```python
from build123d import *

# Parameters (mm, degrees)
SKETCH1_W           = 18
SKETCH1_H           = 13
SKETCH1_R           = 0.5
SKETCH1_R_2         = 1.5
BOSS_EXTRUDE1_DEPTH = 1.5
SKETCH2_W           = 1.829914293
SKETCH2_H           = 3.482740107
BOSS_EXTRUDE2_DEPTH = 1.75
SKETCH3_W           = 4.928962693
SKETCH3_H           = 2.951474666
SKETCH3_W_2         = 1.003501387
SKETCH3_H_2         = 2.331664987
SKETCH3_W_3         = 0.8854424
SKETCH3_W_4         = 0.944471893
SKETCH3_H_3         = 2.095547014
SKETCH3_W_5         = 0.914957147
SKETCH3_H_4         = 2.213606
SKETCH3_W_6         = 2.420209226
SKETCH3_H_5         = 0.914957147
SKETCH3_W_7         = 2.331664986
SKETCH3_W_8         = 2.066032267
SKETCH3_W_9         = 0.79689816
SKETCH3_W_10        = 2.774386186
SKETCH3_H_6         = 2.184091253
SKETCH3_W_11        = 1.741370054
SKETCH3_W_12        = 1.534766827
BOSS_EXTRUDE3_DEPTH = 0.75


with BuildPart() as part:
    # Sketch1 → Boss-Extrude1 (new body)
    with BuildSketch(Plane(origin=(0, 0, 0), x_dir=(1, 0, 0), z_dir=(0, 1, 0))):
        with Locations((9, -6.5)):
            Rectangle(SKETCH1_W, SKETCH1_H)
        with Locations((1.38, -1.38)):
            Circle(SKETCH1_R, mode=Mode.SUBTRACT)
        with Locations((3.92, -1.38)):
            Circle(SKETCH1_R, mode=Mode.SUBTRACT)
        with Locations((6.46, -1.38)):
            Circle(SKETCH1_R, mode=Mode.SUBTRACT)
        with Locations((9, -1.38)):
            Circle(SKETCH1_R, mode=Mode.SUBTRACT)
        with Locations((11.54, -1.38)):
            Circle(SKETCH1_R, mode=Mode.SUBTRACT)
        with Locations((14.08, -1.38)):
            Circle(SKETCH1_R, mode=Mode.SUBTRACT)
        with Locations((16.62, -1.38)):
            Circle(SKETCH1_R, mode=Mode.SUBTRACT)
        with Locations((2.63, -10.37)):
            Circle(SKETCH1_R_2, mode=Mode.SUBTRACT)
    extrude(amount=-BOSS_EXTRUDE1_DEPTH)

    # Sketch2 → Boss-Extrude2 (add)
    with BuildSketch(Plane(origin=(0, 0, 0), x_dir=(1, 0, 0), z_dir=(0, 1, 0))):
        with Locations((13.279638267, -10.115556466)):
            Rectangle(SKETCH2_W, SKETCH2_H)
    extrude(amount=BOSS_EXTRUDE2_DEPTH)

    # Sketch3 → Boss-Extrude3 (add)
    with BuildSketch(Plane(origin=(0, 0, 0), x_dir=(1, 0, 0), z_dir=(0, 1, 0))):
        with Locations((9.368934334, -10.08604172)):
            Rectangle(SKETCH3_W, SKETCH3_H)
        with Locations((1.355680614, -4.492997226)):
            Rectangle(SKETCH3_W_2, SKETCH3_H_2)
        with Locations((2.860932694, -4.492997226)):
            Rectangle(SKETCH3_W_2, SKETCH3_H_2)
        with Locations((4.454729013, -4.492997226)):
            Rectangle(SKETCH3_W_3, SKETCH3_H_2)
        with Locations((6.048525334, -4.492997226)):
            Rectangle(SKETCH3_W_4, SKETCH3_H_2)
        with Locations((6.048525334, -7.56253088)):
            Rectangle(SKETCH3_W_4, SKETCH3_H_3)
        with Locations((7.745623267, -6.027764053)):
            Rectangle(SKETCH3_W_5, SKETCH3_H_4)
        with Locations((8.73436728, -3.784643307)):
            Rectangle(SKETCH3_W_6, SKETCH3_H_5)
        with Locations((12.05477628, -3.784643307)):
            Rectangle(SKETCH3_W_7, SKETCH3_H_5)
        with Locations((15.847421227, -3.784643307)):
            Rectangle(SKETCH3_W_8, SKETCH3_H_5)
        with Locations((13.619057853, -6.027764053)):
            Rectangle(SKETCH3_W_9, SKETCH3_H_4)
        with Locations((15.965480213, -6.927963827)):
            Rectangle(SKETCH3_W_10, SKETCH3_H_6)
        with Locations((16.009752333, -10.277887574)):
            Rectangle(SKETCH3_W_11, SKETCH3_H_5)
        with Locations((10.711855307, -6.027764053)):
            Rectangle(SKETCH3_W_12, SKETCH3_H_4)
    extrude(amount=BOSS_EXTRUDE3_DEPTH)


solid = part.part
```
Part model, mm, in its own coordinate system. A direction names the side the tool comes from. Coordinates: 2 decimals unless noted, no trailing zeros. Order: outer loops, then holes, each group sorted by start corner. A loop starts at its lowest first (then second) coordinate and runs counter-clockwise, first axis right, second up. Notation, with made-up numbers: (-9.5, -17.75) -> (0.5, -17.75) arc R18 cw to (0.5, 6.25) -> close; hole circle Ø3 at (74.25, 50). An arc over 180 degrees is marked (long way). Put each result on its own line as item: value. Start each with the question number.
(1) Probe line 1 along Z through (x, y) = (2.63, -0.9); line 2 along Z through (x, y) = (6.46, -1.15); line 3 along Y through (x, z) = (8.5, 5). List the from-to ranges inside material, lowest first. Write a range as [from, to].
(2) Band-saw the part on A-A (x = 16.62). Give the cut face in (y, z), then the cut area to 3 significant figures.
(3) Mould opens along Z. For faces 5 (the face through (13, 1, 8.374)), 6 (the face through (4.4, 0.75, 4.5)), 7 (the face through (9, -1, 0)) say: pulls with the +Z half, pulls with the -Z half, needs draft (parallel to the pull), parting line crosses it, or undercut.
(4) Band-saw the part on D-D (x = 1.38). Give the cut face in (y, z).
(5) Band-saw the part on B-B (z = 1.38). Count the separate pieces of the cut face and the enclosed holes in it, then the cut area to 3 significant figures.
(6) Which spindle directions (+Z, -Z, +X, -X, +Y, -Y) get a long thin tool onto all of the face, cutting with end or side? Do faces 1 (the face through (12, 0.75, 4)), 2 (the face through (16, 0.75, 10)), 3 (the face through (12.365, 1, 10)), 4 (the face through (9, 0.75, 4)). Say none if no direction does.
(7) Pin check, flat tips, straight feed: pin 1 Ø0.8 at (y, z) = (0.5, 4) entering from +X; pin 2 Ø0.6 at (x, y) = (6, 0.5) entering from -Z; pin 3 Ø0.8 at (x, y) = (3, 0.5) entering from +Z. Stop position of each tip, or through.
Determined:
1. line 1: z = [0, 8.87], [11.87, 13]
1. line 2: z = [0, 0.88], [1.88, 13]
1. line 3: y = [-1.5, 0]
2. outline: (-1.5, 0) -> (0, 0) -> (0, 0.88) -> (-1.5, 0.88) -> close; (-1.5, 1.88) -> (0, 1.88) -> (0, 3.33) -> (0.75, 3.33) -> (0.75, 4.24) -> (0, 4.24) -> (0, 5.84) -> (0.75, 5.84) -> (0.75, 8.02) -> (0, 8.02) -> (0, 9.82) -> (0.75, 9.82) -> (0.75, 10.74) -> (0, 10.74) -> (0, 13) -> (-1.5, 13) -> close
2. area: 21.0 mm²
3. face 5: undercut
3. face 6: needs draft
3. face 7: pulls with the -Z half
4. outline: (-1.5, 0) -> (0, 0) -> (0, 0.88) -> (-1.5, 0.88) -> close; (-1.5, 1.88) -> (0, 1.88) -> (0, 3.33) -> (0.75, 3.33) -> (0.75, 5.66) -> (0, 5.66) -> (0, 9.54) -> (-1.5, 9.54) -> close; (-1.5, 11.2) -> (0, 11.2) -> (0, 13) -> (-1.5, 13) -> close
5. separate pieces: 8
5. enclosed holes: 0
5. area: 16.5 mm²
6. face 1: -Z, +X, -X, +Y
6. face 2: +Z, -Z, +X, +Y
6. face 3: +Z, +Y
6. face 4: +Z, -Z, +X, -X, +Y
7. pin 1: stops at x = 16.88
7. pin 2: stops at z = 3.33
7. pin 3: stops at z = 5.66
